from build123d import *

# Parameters (mm, degrees)
SKETCH1_W           = 390
SKETCH1_H           = 90
BOSS_EXTRUDE1_DEPTH = 5
SKETCH2_R           = 1.25
CUT_EXTRUDE1_DEPTH  = 15
SKETCH3_R           = 1.25
CUT_EXTRUDE2_DEPTH  = 15
CUT_EXTRUDE3_START  = -15
SKETCH4_R           = 1.25
CUT_EXTRUDE3_DEPTH  = 15


with BuildPart() as part:
    # Sketch1 → Boss-Extrude1 (new body)
    with BuildSketch(Plane.XY):
        with Locations((195, 45)):
            Rectangle(SKETCH1_W, SKETCH1_H)
    extrude(amount=BOSS_EXTRUDE1_DEPTH)

    # Sketch2 → Cut-Extrude1 (cut)
    with BuildSketch(Plane.ZY):
        with Locations((2.5, 45)):
            Circle(SKETCH2_R)
    extrude(amount=-CUT_EXTRUDE1_DEPTH, mode=Mode.SUBTRACT)

    # Sketch3 → Cut-Extrude2 (cut)
    with BuildSketch(Plane(origin=(0, 0, 0), x_dir=(-1, 0, 0), z_dir=(0, -1, 0))):
        with Locations(Location((-35, -2.5, 0), (0, 0, 90))):
            Circle(SKETCH3_R)
        with Locations(Location((-355, -2.5, 0), (0, 0, 90))):
            Circle(SKETCH3_R)
    extrude(amount=-CUT_EXTRUDE2_DEPTH, mode=Mode.SUBTRACT)

    # Sketch4 → Cut-Extrude3 (cut)
    with BuildSketch(Plane(origin=(390, 0, 0), x_dir=(0, 0, -1), z_dir=(1, 0, 0)).offset(CUT_EXTRUDE3_START)):
        with Locations(Location((-2.5, 45, 0), (0, 0, 180))):
            Circle(SKETCH4_R)
    extrude(amount=CUT_EXTRUDE3_DEPTH, mode=Mode.SUBTRACT)


solid = part.part
Geometry check sheet. Reference: the model listing, model coordinates, mm. Give positions to 0.01 mm unless a question says otherwise; leave off trailing zeros. Put each result on its own line as item: value.
1. Draft check along Z on faces 1 (the flat face through (192, 46, 5)), 2 (the flat face through (192, 46, 0)). Enter one of: +Z half, -Z half, draft (parallel to the pull), parting line (faces both ways), or undercut.
Ans:
face 1: +Z half
face 2: -Z half
2. Thickness scan on line 1 (X direction, y = 4.5, z = 2.5); line 2 (Z direction, x = 355, y = 7); line 3 (Y direction, x = 5.5, z = 2.5). Record the ranges inside material, lowest first.
Ans:
line 1: x = 0 to 33.75, 36.25 to 353.75, 356.25 to 390
line 2: z = 0 to 1.25, 3.75 to 5
line 3: y = 0 to 43.75, 46.25 to 90
3. Go/stop test with flat-tipped pins: pin 1 (1.2 mm diameter, centred on y = 45, z = 3, fed in from +X); pin 2 (0.8 mm diameter, centred on x = 355.5, z = 2.5, fed in from -Y); pin 3 (2 mm diameter, centred on y = 45, z = 2.5, fed in from -X). Record where each tip stops, or that it passes through.
Ans:
pin 1: stops at x = 375
pin 2: stops at y = 15
pin 3: stops at x = 15
